Design review of the part built by this model. Coordinates are the model's own, in mm. A direction names the side the tool comes from. Coordinates: 2 decimals unless noted, no trailing zeros. Loops run counter-clockwise (first coordinate to the right, second up) from the corner with the lowest first, then second, coordinate; pieces in that order, holes last. Notation, with made-up numbers: (18.25, 70.5) -> (68.25, 70.5) arc R22 cw to (68.25, 91.5) -> close; hole circle Ø1 at (18, 27). An arc over 180 degrees is marked (long way). One line per item, written item: value. Start each with the question number.
1. Machinability: for faces 5 (the flat face through (-1, -1, 20)), 6 (the flat face through (-15, -2, 13)), which of the approach directions +Z, -Z, +X, -X, +Y, -Y give a long, thin tool a straight path to every point of the face, cutting with its end or side? Answer none if there is none.
2. Add section C-C on z = 10. Write out the cut boundary in (x, y) (3 decimals).
3. Add section A-A on y = 0. Write out the cut boundary in (x, z) (3 decimals), plus the area to 3 significant figures.
4. For probe 1 along Z at (x, y) = (-21, -11); probe 2 along Z at (x, y) = (11.5, 7.5); probe 3 along X at (y, z) = (-11, 17.5) (3 decimals), list the stretches that pass through material, from the lowest coordinate up.
5. Add section D-D on y = 17.5. Write out the cut boundary in (x, z) (3 decimals), plus the area to 3 significant figures.
6. Add section B-B on x = -11. Write out the cut boundary in (y, z).
7. Draft analysis for pull direction Z (two halves, no side actions). For faces 1 (the flat face through (-20, 27.25, 0)), 2 (the flat face through (10, -19, 18)), 3 (the flat face through (1, -2, -20)), 4 (the flat face through (10, 19, 18)), state which applies: pulls with the +Z half, pulls with the -Z half, needs draft (parallel to the pull), parting line crosses it, or undercut.
8. Insertion check: pin 1 (10 mm diameter, centred on x = 17, z = 12, fed in from +Y); pin 2 (9.5 mm diameter, centred on x = 4.5, z = 7.5, fed in from +Y). Each pin has a flat end and moves straight along its axis. Give the tip position at first contact, or say it passes through.
Autodesk Inventor part; units mm, degrees
ref_plane "YZ Plane" through (0, 0, 0) normal (1, 0, 0) x (0, 1, 0)
ref_plane "XZ Plane" through (0, 0, 0) normal (0, 1, 0) x (-1, 0, 0)
ref_plane "XY Plane" through (0, 0, 0) normal (0, 0, 1) x (1, 0, 0)
sketch "Sketch1" plane through (0, 0, 0) normal (0, 0, 1) x (1, 0, 0)
  circle A0 centre (-16.125, 0) radius 6
  arc A1 (16.125, -18.735) -> (5.2413, -15.2494) centre (10.125, -18.735) ccw
  arc A2 (16.125, 18.735) -> (5.2413, 15.2494) centre (10.125, 18.735) ccw
  circle A3 centre (10.125, 18.735) radius 7.5
  circle A4 centre (10.125, -18.735) radius 7.5
  line L0 (16.125, 27.25) -> (-16.125, 27.25)
  arc A5 (-16.125, 27.25) -> (-16.125, -27.25) centre (-16.125, 0) ccw
  line L1 (-16.125, -27.25) -> (16.125, -27.25)
  arc A6 (16.125, -27.25) -> (16.125, 27.25) centre (16.125, 0) ccw
  arc A7 (-29.2589, 27.25) -> (-16.125, -30.25) centre (-16.125, 0) ccw
  line L2 (-16.125, -30.25) -> (16.125, -30.25)
  arc A8 (16.125, -30.25) -> (29.2589, 27.25) centre (16.125, 0) ccw
  line L3 (-16.125, -30.25) -> (16.125, -30.25)
  line L4 (46.375, -30.25) -> (46.375, 27.25)
  line L5 (-46.375, 27.25) -> (-46.375, -30.25)
  line L6 (-46.375, -30.25) -> (46.375, 30.25) construction
  line L7 (46.375, -30.25) -> (-46.375, 30.25) construction
  line L8 (46.375, 27.25) -> (-46.375, 27.25)
  line L9 (-16.125, -30.25) -> (16.125, -30.25)
  line L10 (46.375, -30.25) -> (46.375, -32.25)
  line L11 (46.375, -32.25) -> (-46.375, -32.25)
  line L12 (-46.375, -32.25) -> (-46.375, -30.25)
  line L13 (-46.375, 27.25) -> (46.375, 27.25)
  line L14 (46.375, 27.25) -> (46.375, -32.25)
  line L15 (46.375, -32.25) -> (-46.375, -32.25)
  line L16 (-46.375, -32.25) -> (-46.375, 27.25)
  point P0 (0, 0)
  point P1 (0, 26.25)
  point P2 (0, -26.25)
  dimension "d1" = 12
  dimension "d3" = 12
  dimension "d4" = 12
  dimension "d6" = 15
  dimension "d7" = 15
  dimension "d9" = 3
  dimension "d12" = 2
extrude "Extrusion2" add sketch "Sketch1" along normal mid plane 40 contours A0 | A3 | A4 | A6 L1 A5 L0 | L8 A8 L2 A7 A5 L1 A6 | L8 L4 A8 | A7 L5 L8 | L4 L10 L11 L12 L5 A7 L2 A8
extrude "Extrusion3" cut sketch "Sketch1" along normal mid plane 36 contours A6 L1 A5 L0
extrude "Extrusion4" cut sketch "Sketch1" along normal mid plane 36 contours A0 | A3 | A4
sketch "Sketch2" plane through (0, 0, 20) normal (0, 0, 1) x (1, 0, 0)
  arc A0 (16.125, -18.735) -> (5.2413, -15.2494) centre (10.125, -18.735) ccw
  circle A1 centre (10.125, 18.735) radius 7.5
  circle A2 centre (-16.125, 0) radius 6
  circle A3 centre (10.125, 18.735) radius 7.5
  circle A4 centre (10.125, 18.735) radius 10.5
  circle A5 centre (10.125, -18.735) radius 7.5
  circle A6 centre (10.125, -18.735) radius 10.5
  circle A7 centre (-16.125, 0) radius 1.65
  circle A8 centre (-16.125, 0) radius 3.5
  point P0 (0, 0)
  point P1 (16.125, 0)
  dimension "d19" = 21
  dimension "d20" = 15
  dimension "d21" = 21
  dimension "d22" = 3.3
  dimension "d23" = 7
extrude "Extrusion5" add sketch "Sketch2" against normal blind 7 contours A4 | A6 | A8
sketch "Sketch3" plane through (0, 0, -20) normal (0, 0, -1) x (-1, 0, 0)
  circle A0 centre (-16.125, 0) radius 8.1
  circle A1 centre (-16.125, 0) radius 11.1
  point P0 (0, 0)
  dimension "d26" = 16.2
  dimension "d27" = 3
extrude "Extrusion6" add sketch "Sketch3" against normal blind 5
extrude "Extrusion7" cut sketch "Sketch3" against normal blind 5 contours A0
properties part number "referencia"
Worked answers:
1. face 5: +Z, +X, -X, +Y, -Y
1. face 6: none
2. outline: (-46.375, -32.25) -> (46.375, -32.25) -> (46.375, 27.25) -> (16.125, 27.25) arc R27.25 cw to (16.125, -27.25) -> (-16.125, -27.25) arc R27.25 cw to (-16.125, 27.25) -> (-46.375, 27.25) -> close
3. outline: (-46.375, -20) -> (8.025, -20) -> (8.025, -15) -> (5.025, -15) -> (5.025, -18) -> (-43.375, -18) -> (-43.375, 18) -> (-19.625, 18) -> (-19.625, 13) -> (-17.775, 13) -> (-17.775, 18) -> (-14.475, 18) -> (-14.475, 13) -> (-12.625, 13) -> (-12.625, 18) -> (43.375, 18) -> (43.375, -18) -> (27.225, -18) -> (27.225, -15) -> (24.225, -15) -> (24.225, -20) -> (46.375, -20) -> (46.375, 20) -> (-46.375, 20) -> close
3. area: 591 mm²
4. probe 1: z = -20 to -18, 18 to 20
4. probe 2: z = -20 to -15, 18 to 20
4. probe 3: x = -46.375 to -41.056, 3.024 to 17.226, 41.056 to 46.375
5. outline: (-46.375, -20) -> (46.375, -20) -> (46.375, 20) -> (-46.375, 20) -> close; hole (-37.013, -18) -> (37.013, -18) -> (37.013, 18) -> (20.552, 18) -> (20.552, 13) -> (17.523, 13) -> (17.523, 18) -> (2.727, 18) -> (2.727, 13) -> (-0.302, 13) -> (-0.302, 18) -> (-37.013, 18) -> close
5. area: 1,080 mm²
6. outline: (-32.25, -20) -> (27.25, -20) -> (27.25, -18) -> (-27.25, -18) -> (-27.25, 18) -> (27.25, 18) -> (27.25, 20) -> (-32.25, 20) -> close
7. face 1: needs draft
7. face 2: undercut
7. face 3: pulls with the -Z half
7. face 4: undercut
8. pin 1: stops at y = 29.05
8. pin 2: stops at y = -27.25
